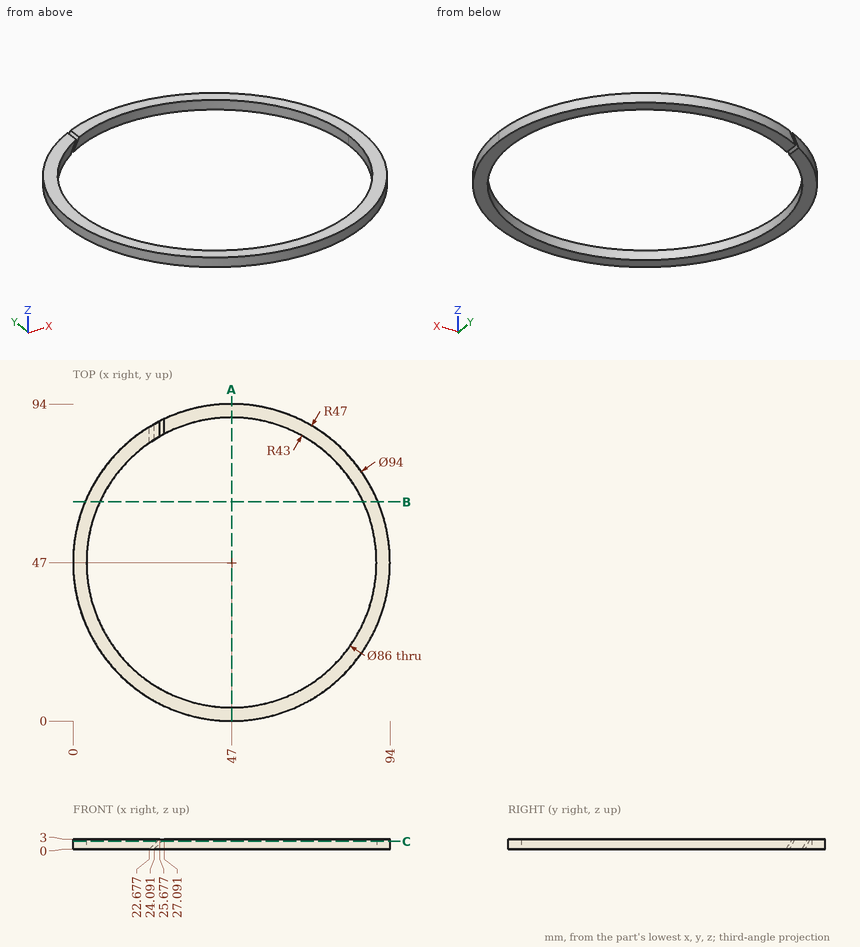
The figure shows three views and two pictorial views of one solid part (mm, origin at its lowest corner). Answer the questions. Coordinates: 2 decimals unless noted, no trailing zeros. Loops run counter-clockwise (first coordinate to the right, second up) from the corner with the lowest first, then second, coordinate; pieces in that order, holes last. Notation, with made-up numbers: (-28.75, 48) -> (-6.75, 48) arc R19 ccw to (-6.75, 64) -> close; hole circle Ø6 at (80, 76.25). An arc over 180 degrees is marked (long way). Use one line per item in the form item = value. Start each with the question number.
Item 1: The part is cut by section A-A on x = 47. Determine the outline of the cut face in (y, z).
Item 2: The part is cut by section C-C on z = 2.3. Determine the outline of the cut face in (x, y), then the cut area to 3 significant figures.
Item 3: A flat-ended cylindrical pin translates along its axis: pin 1 Ø1 at (x, z) = (10, 2) entering from -Y. Find the tip coordinate at first contact, or state that the pin passes through.
Item 4: Consider L1, parallel to Y at x = 47, z = 1.1; L2, parallel to Y at x = 26, z = 1.8. Determine where each line is inside the solid, lowest interval first. Write a range as [from, to].
Item 5: The part is cut by section B-B on y = 65. Determine the outline of the cut face in (x, z), then the cut area to 3 significant figures.
Answer key:
q1.outline = (0, 0) -> (4, 0) -> (4, 3) -> (0, 3) -> close; (90, 0) -> (94, 0) -> (94, 3) -> (90, 3) -> close
q2.outline = (24.98, 83.93) -> (24.98, 88.52) arc R47 ccw (long way) to (26.39, 89.24) -> (26.39, 84.74) arc R43 cw (long way) to start
q2.area = 1,120 mm2
q3.pin_1 = 17.39
q4.L1 = [0, 4], [90, 94]
q4.L2 = [4.95, 9.48], [84.52, 89.05]
q5.outline = (3.58, 0) -> (7.95, 0) -> (7.95, 3) -> (3.58, 3) -> close; (86.05, 0) -> (90.42, 0) -> (90.42, 3) -> (86.05, 3) -> close
q5.area = 26.2 mm2
